```python
from build123d import *

# Parameters (mm, degrees)
SKETCH1_W           = 74
SKETCH1_H           = 48
SKETCH1_W_2         = 5
SKETCH1_H_2         = 5
BOSS_EXTRUDE1_DEPTH = 3
BOSS_EXTRUDE2_START = -1
SKETCH1_4_W         = 71.4
SKETCH1_4_H         = 45.4
SKETCH1_4_W_2       = 5
SKETCH1_4_H_2       = 5
BOSS_EXTRUDE2_DEPTH = 1
CHAMFER1_SIZE       = 1


with BuildPart() as part:
    # Sketch1 → Boss-Extrude1 (new body)
    with BuildSketch(Plane(origin=(0, 0, 0), x_dir=(1, 0, 0), z_dir=(0, 1, 0))):
        Rectangle(SKETCH1_W, SKETCH1_H)
        with Locations((-25, 0)):
            Rectangle(SKETCH1_W_2, SKETCH1_H_2, mode=Mode.SUBTRACT)
    extrude(amount=BOSS_EXTRUDE1_DEPTH)

    # Sketch1<4> → Boss-Extrude2 (add)
    with BuildSketch(Plane(origin=(0, 0, 0), x_dir=(1, 0, 0), z_dir=(0, 1, 0)).offset(BOSS_EXTRUDE2_START)):
        Rectangle(SKETCH1_4_W, SKETCH1_4_H)
        with Locations((-25, 0)):
            Rectangle(SKETCH1_4_W_2, SKETCH1_4_H_2, mode=Mode.SUBTRACT)
    extrude(amount=BOSS_EXTRUDE2_DEPTH)

    # Chamfer1
    chamfer1_edges = [part.edges().sort_by_distance(p)[0] for p in [
        (0, 3, 24),
        (37, 3, 0),
        (0, 3, -24),
        (-37, 3, 0),
    ]]
    chamfer(chamfer1_edges, length=CHAMFER1_SIZE)


solid = part.part
```
Build history of the part. All positions in model axes, mm. A direction names the side the tool comes from. Coordinates: 2 decimals unless noted, no trailing zeros. Write each loop counter-clockwise with the first axis right and the second up, starting at its lowest first coordinate (ties: lowest second). Pieces come first, ordered by that corner, then holes.
1. Band-saw the part on B-B, the plane x = -14. Give the cut face in (y, z), and give its area (3 significant figures).
Answer block:
outline: (-1, -22.7) - (0, -22.7) - (0, -24) - (2, -24) - (3, -23) - (3, 23) - (2, 24) - (0, 24) - (0, 22.7) - (-1, 22.7) - close
area: 188 mm2
2. Drill centre lines: probe 1 along X at (y, z) = (-0.5, 1); probe 2 along Z at (x, y) = (-25, 1.2); probe 3 along X at (y, z) = (-0.5, 8). Where is each one in solid material? Low to high.
Answer block:
probe 1: x = -35.7 to -27.5, -22.5 to 35.7
probe 2: z = -24 to -2.5, 2.5 to 24
probe 3: x = -35.7 to 35.7
3. Band-saw the part on A-A, the plane x = -24.5. Give the cut face in (y, z), and give its area (3 significant figures).
Answer block:
outline: (-1, -22.7) - (0, -22.7) - (0, -24) - (2, -24) - (3, -23) - (3, -2.5) - (-1, -2.5) - close; (-1, 2.5) - (3, 2.5) - (3, 23) - (2, 24) - (0, 24) - (0, 22.7) - (-1, 22.7) - close
area: 168 mm2
4. 3-axis set-ups, long thin cutter, end or side, ignore diameter. For faces 4 (the flat face through (-1, 1, -24)), 5 (the flat face through (-25, 1, 2.5)): which of +Z, -Z, +X, -X, +Y, -Y reach the whole face in a straight line?
Answer block:
face 4: -Z, +X, -X, +Y, -Y
face 5: +Y, -Y
5. Pull direction X, two halves, no side cores. Call faces 1 (the flat face through (0, -1, 0)), 2 (the flat face through (37, 1, 0)), 3 (the flat face through (-27.5, 1, 0)): released by +X, released by -X, zero draft, split by the parting line, or undercut.
Answer block:
face 1: zero draft
face 2: released by +X
face 3: undercut
6. Drop flat-ended pins along their axis: pin 1 (0.8 mm diameter, centred on y = -0.5, z = 7, fed in from -X); pin 2 (0.5 mm diameter, centred on x = 0.5, y = -0.5, fed in from +Z). Give the stop position or say it passes through.
Answer block:
pin 1: stops at x = -35.7
pin 2: stops at z = 22.7
